Geometry: final body of the model. Coordinates: model frame, mm. Face numbers are marked on the shaded views. A direction names the side the tool comes from. Give positions to 0.01 mm unless a question says otherwise; leave off trailing zeros. Order: outer loops, then holes, each group sorted by start corner. A loop starts at its lowest first (then second) coordinate and runs counter-clockwise, first axis right, second up. Notation, with made-up numbers: M 16,56.25 L 47,56.25 A30 cw 47,90.25 Z; hole C 44.5,9 d3. An arc over 180 degrees is marked long. Use CSV: the item, a comma, the result in double quotes.
```python
from build123d import *

# Parameters (mm, degrees)
SKETCH_1_R          = 3
EXTRUDE_1_DEPTH     = 2.5
CUT_EXTRUDE_START   = -2.5
CUT_EXTRUDE_2_DEPTH = 2.5
CUT_EXTRUDE_START_2 = -20
CUT_EXTRUDE_3_DEPTH = 20
FILLET_2_R          = 1.5


with BuildPart() as part:
    # 草图1 → 凸台-拉伸1 (new body)
    with BuildSketch(Plane.XY):
        with BuildLine():
            ThreePointArc((0.416666667, 4.982608643), (-4.995650269, 0.20851473), (0, -5))
            Line((0, -5), (19.972590695, -6.046719125))
            Line((19.972590695, -6.046719125), (25.587337922, -2.545654792))
            ThreePointArc((25.587337922, -2.545654792), (26.916096314, 0.704544029), (24.25, 2.989565186))
            Line((24.25, 2.989565186), (0.416666667, 4.982608643))
        make_face()
        Circle(SKETCH_1_R, mode=Mode.SUBTRACT)
        with BuildLine():
            ThreePointArc((9, -1.3), (7.7, 0), (9, 1.3))
            Line((9, 1.3), (24, 1.3))
            ThreePointArc((24, 1.3), (25.3, 0), (24, -1.3))
            Line((24, -1.3), (9, -1.3))
        make_face(mode=Mode.SUBTRACT)
    extrude(amount=EXTRUDE_1_DEPTH)

    # 草图2 → 切除-拉伸2 (cut)
    with BuildSketch(Plane.XY.offset(2.5).offset(CUT_EXTRUDE_START)):
        with BuildLine():
            Line((24.851438624, -3.004523319), (25.587337922, -2.545654792))
            ThreePointArc((25.587337922, -2.545654792), (26.931709032, -0.636460643), (26.5, 1.658312395))
            Line((26.5, 1.658312395), (24.851438624, -3.004523319))
        make_face()
    extrude(amount=CUT_EXTRUDE_2_DEPTH, mode=Mode.SUBTRACT)

    # 草图3 → 切除-拉伸3 (cut)
    with BuildSketch(Plane.XY.offset(2.5).offset(CUT_EXTRUDE_START_2)):
        with BuildLine():
            ThreePointArc((-4.900680589, -0.991629852), (-3.165584523, -3.87028095), (0, -5))
            Line((0, -5), (3.814269781, -5.199897409))
            ThreePointArc((3.814269781, -5.199897409), (-0.9669941, -3.973392585), (-4.900680589, -0.991629852))
        make_face()
    extrude(amount=CUT_EXTRUDE_3_DEPTH, mode=Mode.SUBTRACT)

    # 圆角2
    fillet_2_edges = [part.edges().sort_by_distance(p)[0] for p in [
        (19.972590695, -6.046719125, 1.25),
        (26.5, 1.658312395, 1.25),
        (24.851438624, -3.004523319, 1.25),
        (-4.900680589, -0.991629852, 1.25),
    ]]
    fillet(fillet_2_edges, radius=FILLET_2_R)


solid = part.part
```
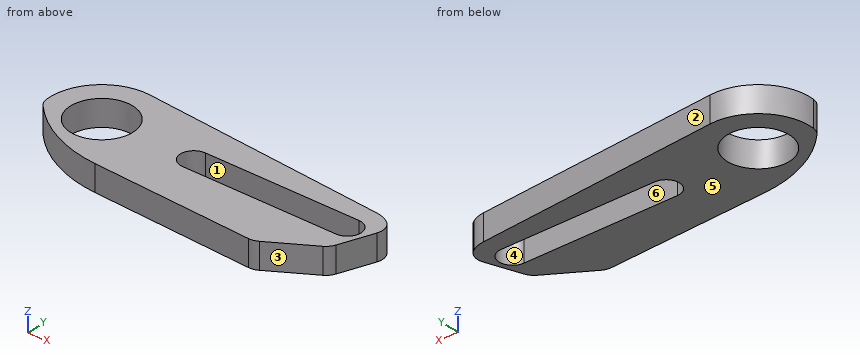
1. Line query: line 1 (X direction, y = -0.25, z = 0.2); line 2 (X direction, y = 0.25, z = 1.7); line 3 (Y direction, x = 0, z = 0.75). Output: solid intervals per line, ascending.
Answer:
line 1,"-4.99 to -2.99, 2.99 to 7.72, 25.28 to 25.83"
line 2,"-4.99 to -2.99, 2.99 to 7.72, 25.28 to 26"
line 3,"-4.39 to -3, 3 to 5"
2. Pin query (flat end, axial travel): pin 1 Ø1.5 at (x, y) = (20, -1) entering from -Z; pin 2 Ø1.5 at (x, z) = (2.5, 1) entering from -Y; pin 3 Ø5.5 at (x, y) = (0, 0) entering from -Z. Return the tip coordinate at first contact, or that it passes through.
Answer:
pin 1,"z = 0"
pin 2,"y = -5.16"
pin 3,"through"
3. Section B-B, the plane x = 1. Return the cut outline in (y, z).
Answer:
outline,"M -4.73,0 L -2.83,0 L -2.83,2.5 L -4.73,2.5 Z; M 2.83,0 L 4.93,0 L 4.93,2.5 L 2.83,2.5 Z"
4. Pull-direction query (X, two-part tool) for the marked faces 3, 4, 5 and 6; classes: +X half, -X half, draft (parallel to the pull), parting line (faces both ways), or undercut.
Answer:
face 3,"+X half"
face 4,"undercut"
face 5,"draft"
face 6,"undercut"
5. Section C-C, the plane z = 2.2. Give the number of separate pieces and of enclosed holes in the cut face, plus the area to 3 significant figures.
Answer:
separate pieces,"1"
enclosed holes,"2"
area,"197 mm2"
6. Section A-A, the plane y = 0. Return the cut outline in (x, z).
Answer:
outline,"M -5,0 L -3,0 L -3,2.5 L -5,2.5 Z; M 3,0 L 7.7,0 L 7.7,2.5 L 3,2.5 Z; M 25.3,0 L 25.91,0 L 25.91,2.5 L 25.3,2.5 Z"
7. Section D-D, the plane x = 16. Return the cut outline in (y, z).
Answer:
outline,"M -5.84,0 L -1.3,0 L -1.3,2.5 L -5.84,2.5 Z; M 1.3,0 L 3.68,0 L 3.68,2.5 L 1.3,2.5 Z"
8. Reachability of the marked faces 1 and 2 from +Z, -Z, +X, -X, +Y, -Y: full face, straight path, thin tool, end or side. Return the list, or none.
Answer:
face 1,"+Z, -Z"
face 2,"+Z, -Z, +X, +Y"
